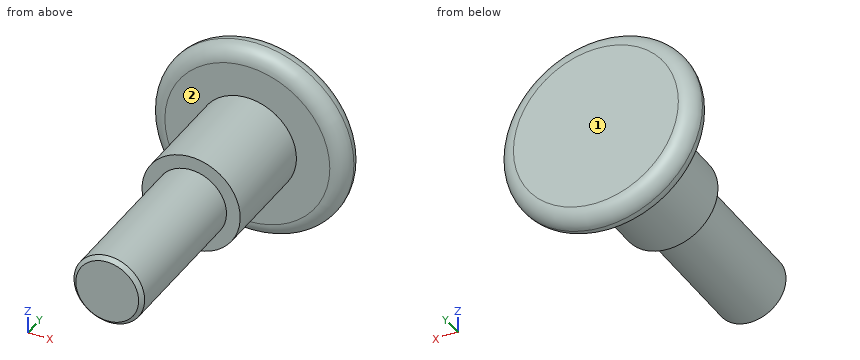
```python
from build123d import *

# Parameters (mm, degrees)
FILETE2_R     = 2
CHANFRO1_SIZE = 0.5


with BuildPart() as part:
    # Esboço1 → Revolução1 (revolve)
    with BuildSketch(Plane.XY, mode=Mode.PRIVATE) as revolu_o1_sk:
        Polygon((0, 56.545238095), (12.5, 56.545238095), (12.5, 52.545238095), (6.25, 52.545238095), (6.25, 39.145238095), (4.5, 39.145238095), (4.5, 19.145238095), (0, 19.145238095), align=None)
    revolve(revolu_o1_sk.sketch.rotate(Axis((0, -62.761627907, 0), (0, 1, 0)), 90), axis=Axis((0, -62.761627907, 0), (0, 1, 0)))

    # Filete2
    filete2_edges = [part.edges().sort_by_distance(p)[0] for p in [
        (0, 52.545238095, 12.5),
        (0, 56.545238095, 12.5),
    ]]
    fillet(filete2_edges, radius=FILETE2_R - 0.0001)  # a hair under: the kernel refuses the full size

    # Chanfro1
    chanfro1_edges = [part.edges().sort_by_distance(p)[0] for p in [
        (0, 19.145238095, 4.5),
    ]]
    chamfer(chanfro1_edges, length=CHANFRO1_SIZE)


solid = part.part
```
The listing builds one solid part. Answer for the finished solid, in the listing's coordinates (mm). Face numbers are marked on the shaded views. A direction names the side the tool comes from. Round coordinates to 2 decimals unless told otherwise and drop trailing zeros. Loops run counter-clockwise (first coordinate to the right, second up) from the corner with the lowest first, then second, coordinate; pieces in that order, holes last.
Q1. Find the intervals of material crossed by line 1 (Y direction, x = 7.75, z = -2.25); line 2 (Y direction, x = 1.25, z = -4.5); line 3 (X direction, y = 38.5, z = -3), in increasing order.
Q2. Which of the six approach directions +Z, -Z, +X, -X, +Y, -Y give full straight-line access (tool end or side, diameter ignored) to the marked faces 1 and 2?
Q3. Given pin 1 Ø3 at (y, z) = (35.5, -4.5) entering from -X; pin 2 Ø1 at (x, z) = (8, -10) entering from +Y; pin 3 Ø3 at (x, y) = (-2.5, 40.5) entering from +Z, each flat-ended and moving along its own axis, determine where each tip first touches the part or whether it passes through.
Q4. Section D-D, the plane y = 45.5 is taken. Determine the outline of the cut face in (x, z).
Q5. Section C-C, the plane y = 28.5 is taken. Determine the outline of the cut face in (x, z), then the cut area to 3 significant figures.
Completed:
1. line 1: y = 52.55 to 56.55
1. line 2: y = 39.15 to 56.55
1. line 3: x = -3.35 to 3.35
2. face 1: +Z, -Z, +X, -X, +Y
2. face 2: -Y
3. pin 1: stops at x = -3.35
3. pin 2: stops at y = 55.4
3. pin 3: stops at z = 6.17
4. outline: circle Ø12.5 at (0, 0)
5. outline: circle Ø9 at (0, 0)
5. area: 63.6 mm2
